```python
from build123d import *

# Parameters (mm, degrees)
CROQUIS1_W              = 57
CROQUIS1_H              = 24.959470006
CROQUIS1_W_2            = 43
CROQUIS1_H_2            = 22
MAIN_DEPTH              = 28
CROQUIS2_W              = 27.955905163
CROQUIS2_H              = 20.987971864
CORTE_CAJA_DEPTH        = 24.95947
CROQUIS3_W              = 32
CROQUIS3_H              = 24.959470006
SALIENTE_EXTRUIR2_DEPTH = 2.25
REDONDEO_LATERALES_R    = 3
CROQUIS7_R              = 1.3
TALADROS_BASE_DEPTH     = 11
CAJEADO_CABLE_DEPTH     = 10
CAJEADO_REDONDEO_R      = 2
CORTAR_EXTRUIR1_DEPTH   = 24.95947


with BuildPart() as part:
    # Croquis1 → Main (new body)
    with BuildSketch(Plane(origin=(0, 0, 0), x_dir=(1, 0, 0), z_dir=(0, 1, 0))):
        with Locations((11.181999645, 13.428246359)):
            Rectangle(CROQUIS1_W, CROQUIS1_H)
        with Locations((10.844499645, 13.430306654)):
            Rectangle(CROQUIS1_W_2, CROQUIS1_H_2, mode=Mode.SUBTRACT)
    extrude(amount=MAIN_DEPTH)

    # Croquis2 → Corte Caja (cut)
    with BuildSketch(Plane.XY.offset(-0.948511356)):
        with Locations((28.659952227, 20.493985932)):
            Rectangle(CROQUIS2_W, CROQUIS2_H)
    extrude(amount=-CORTE_CAJA_DEPTH, mode=Mode.SUBTRACT)

    # Croquis3 → Saliente-Extruir2 (add)
    with BuildSketch(Plane(origin=(0, 28, 0), x_dir=(1, 0, 0), z_dir=(0, 1, 0))):
        with Locations((-1.318000355, 13.428246359)):
            Rectangle(CROQUIS3_W, CROQUIS3_H)
    extrude(amount=SALIENTE_EXTRUIR2_DEPTH)

    # Redondeo Laterales
    redondeo_laterales_edges = [part.edges().sort_by_distance(p)[0] for p in [
        (39.681999645, 5, -25.907981362),
        (39.681999645, 5, -0.948511356),
        (-17.318000355, 15.125, -25.907981362),
        (-17.318000355, 15.125, -0.948511356),
    ]]
    fillet(redondeo_laterales_edges, radius=REDONDEO_LATERALES_R)

    # Croquis7 → Taladros Base (cut)
    with BuildSketch(Plane.XZ):
        with Locations((-13.155500355, -8.448511356)):
            Circle(CROQUIS7_R)
        with Locations((-13.155500355, -18.448511356)):
            Circle(CROQUIS7_R)
        with Locations((34.844499645, -8.448511356)):
            Circle(CROQUIS7_R)
        with Locations((34.844499645, -18.448511356)):
            Circle(CROQUIS7_R)
    extrude(amount=-TALADROS_BASE_DEPTH, mode=Mode.SUBTRACT)

    # Croquis8 → Cajeado cable (cut)
    with BuildSketch(Plane.XZ):
        Polygon((-10.655500355, -17.809410949), (-10.655500355, -9.693483102), (-13.79985022, -11.41721999), (-13.79985022, -15.216689513), align=None)
    extrude(amount=-CAJEADO_CABLE_DEPTH, mode=Mode.SUBTRACT)

    # Cajeado Redondeo
    cajeado_redondeo_edges = [part.edges().sort_by_distance(p)[0] for p in [
        (-13.79985022, 5, -11.41721999),
        (-10.655500355, 5, -9.693483102),
        (-10.655500355, 5, -17.809410949),
        (-13.79985022, 5, -15.216689513),
    ]]
    fillet(cajeado_redondeo_edges, radius=CAJEADO_REDONDEO_R)

    # Croquis10 → Cortar-Extruir1 (cut)
    with BuildSketch(Plane.XY.offset(-0.948511356)):
        Polygon((-18.751407395, 10), (41.252258099, 10), (41.252258099, 38.904482254), (-18.751407395, 38.904482254), (-18.751407395, 38.898632989), align=None)
    extrude(amount=-CORTAR_EXTRUIR1_DEPTH, mode=Mode.SUBTRACT)


solid = part.part
```
The listing builds one solid part. Answer for the finished solid, in the listing's coordinates (mm). A direction names the side the tool comes from. Coordinates: 2 decimals unless noted, no trailing zeros. Loops run counter-clockwise (first coordinate to the right, second up) from the corner with the lowest first, then second, coordinate; pieces in that order, holes last. Notation, with made-up numbers: M 77,24.25 L 105,24.25 A16 ccw 105,36.25 Z; hole C 34.5,70 d4. An arc over 180 degrees is marked long. Answer as CSV lines item,"result". Start each with the question number.
(1) The part is cut by section C-C (y = 4). Give the vertices of the cut face in (x, z).
(2) Find the intervals of material crossed by L1, parallel to Z at x = 27, y = 3; L2, parallel to X at y = 7, z = -7; L3, parallel to Z at x = 34, y = 1.5, in increasing order. Write a range as [from, to].
(3) The part is cut by section D-D (z = -7.75). Give the vertices of the cut face in (x, y), and give its area (3 significant figures).
(4) Given pin 1 (1.6 mm diameter, centred on x = 34.84, z = -8.45, fed in from +Y), flat-ended and moving along its own axis, determine where the tip first touches the part or whether it passes through.
(5) The part is cut by section A-A (z = -21.5). Give the vertices of the cut face in (x, y).
(6) The mould has two halves that part along Z. Classify faces 1 (the cylindrical face through (-16.46, 4.93, -25.01)), 2 (the cylindrical face through (33.886, 4.93, -7.57)), 3 (the flat face through (-17.318, 5, -13)), 4 (the flat face through (-13.8, 5, -13)): pulls with the +Z half, pulls with the -Z half, needs draft (parallel to the pull), parting line crosses it, or undercut.
(7) For faces 5 (the flat face through (-10.656, 5, -5)), 6 (the flat face through (11, 5, -0.949)), determine the directions among +Z, -Z, +X, -X, +Y, -Y from which every point of the face is accessible in a straight line to the end or side of a thin tool.
(8) The part is cut by section B-B (x = -6). Give the vertices of the cut face in (y, z), and give its area (3 significant figures).
Determined:
1,outline,"M -17.32,-22.91 A3 ccw -14.32,-25.91 L 36.68,-25.91 A3 ccw 39.68,-22.91 L 39.68,-3.95 A3 ccw 36.68,-0.95 L -14.32,-0.95 A3 ccw -17.32,-3.95 Z; hole C -13.16,-18.45 d2.6; hole C -13.16,-8.45 d2.6; hole M -13.8,-14.27 A2 ccw -13.07,-15.82 L -11.38,-17.21 A2 cw -10.66,-18.75 L -10.66,-24.43 L 32.34,-24.43 L 32.34,-2.43 L -10.66,-2.43 L -10.66,-8.51 A2 cw -11.69,-10.26 L -12.76,-10.85 A2 ccw -13.8,-12.6 Z; hole C 34.84,-18.45 d2.6; hole C 34.84,-8.45 d2.6"
2,L1,"[-25.91, -24.43], [-2.43, -0.95]"
2,L2,"[-17.32, -10.66], [32.34, 39.68]"
2,L3,"[-25.91, -19.44], [-17.46, -9.44], [-7.46, -0.95]"
3,outline,"M -17.32,0 L -14.25,0 L -14.25,10 L -17.32,10 Z; M -12.06,0 L -10.66,0 L -10.66,10 L -12.06,10 Z; M 32.34,0 L 33.75,0 L 33.75,10 L 32.34,10 Z; M 35.94,0 L 39.68,0 L 39.68,10 L 35.94,10 Z"
3,area,"96.1 mm2"
4,pin 1,"through"
5,outline,"M -17.32,0 L -10.66,0 L -10.66,10 L -17.32,10 Z; M 32.34,0 L 39.68,0 L 39.68,10 L 32.34,10 Z"
6,face 1,"pulls with the -Z half"
6,face 2,"undercut"
6,face 3,"needs draft"
6,face 4,"undercut"
7,face 5,"+Y, -Y"
7,face 6,"+Z, +X, -X, +Y, -Y"
8,outline,"M 0,-25.91 L 10,-25.91 L 10,-24.43 L 0,-24.43 Z; M 0,-2.43 L 10,-2.43 L 10,-0.95 L 0,-0.95 Z"
8,area,"29.6 mm2"
